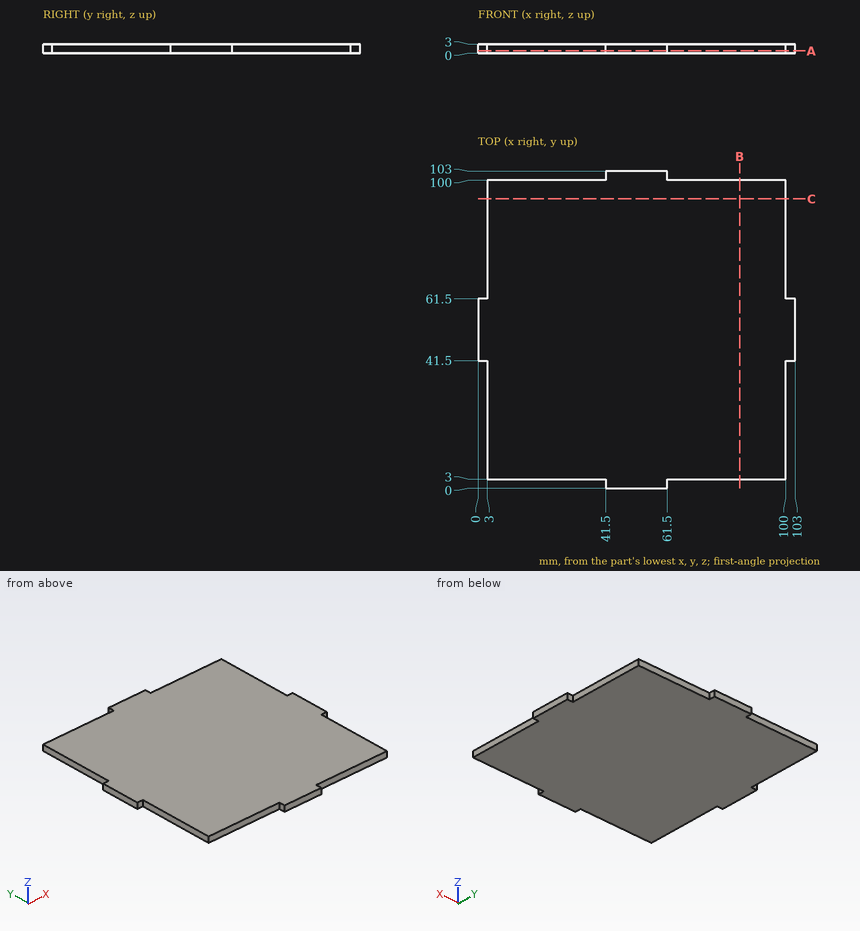
Geometry check sheet. Reference: drawing and pictorial views, mm from the part's lowest x, y, z. Coordinates: 2 decimals unless noted, no trailing zeros. Order: outer loops, then holes, each group sorted by start corner. A loop starts at its lowest first (then second) coordinate and runs counter-clockwise, first axis right, second up.
Item 1: Section check B-B (x = 85). Enter the section's corners in (y, z), plus the area to 3 significant figures.
Item 2: Scan line: line 1 along X through (y, z) = (94, 0.4). Record every from-to range of solid material in increasing order.
Item 3: Depth check by flat-ended pin: pin 1 (1.5 mm diameter, centred on x = 12.5, z = 1.5, fed in from -Y); pin 2 (1.5 mm diameter, centred on x = 1, z = 2, fed in from +Y); pin 3 (1 mm diameter, centred on y = 78, z = 2.5, fed in from +X). Enter the tip coordinate at first touch or a pass-through.
Item 4: Section check A-A (z = 0.8). Enter the section's corners in (x, y), plus the area to 3 significant figures.
Check sheet entries:
1. outline: (3, 0) - (100, 0) - (100, 3) - (3, 3) - close
1. area: 291 mm2
2. line 1: x = 3 to 100
3. pin 1: stops at y = 3
3. pin 2: stops at y = 61.5
3. pin 3: stops at x = 100
4. outline: (0, 41.5) - (3, 41.5) - (3, 3) - (41.5, 3) - (41.5, 0) - (61.5, 0) - (61.5, 3) - (100, 3) - (100, 41.5) - (103, 41.5) - (103, 61.5) - (100, 61.5) - (100, 100) - (61.5, 100) - (61.5, 103) - (41.5, 103) - (41.5, 100) - (3, 100) - (3, 61.5) - (0, 61.5) - close
4. area: 9,650 mm2
